Read the model definition and answer for the solid it produces. Units are mm, in the model's axes. Face numbers are marked on the shaded views. A direction names the side the tool comes from. Give positions to 0.01 mm unless a question says otherwise; leave off trailing zeros. Write each loop counter-clockwise with the first axis right and the second up, starting at its lowest first coordinate (ties: lowest second). Pieces come first, ordered by that corner, then holes. Notation, with made-up numbers: M 73.25,-14.75 L 108.25,-14.75 A23 ccw 108.25,20.25 Z; hole C -2.5,33 d1. An arc over 180 degrees is marked long. Use a Markdown table: item, result. Add a question column.
Item 1: A cutting plane is placed at C-C on x = 0. Count the separate pieces of the cut face and the enclosed holes in it, then the cut area to 3 significant figures.
Item 2: A cutting plane is placed at A-A on z = 47. Determine the outline of the cut face in (x, y), then the cut area to 3 significant figures.
Item 3: A cutting plane is placed at B-B on y = 0. Determine the outline of the cut face in (x, z).
Item 4: Consider probe 1 along Y at (x, z) = (0, -12.5); probe 2 along Y at (x, z) = (10.5, 41.5); probe 3 along Z at (x, y) = (-7, 9). Determine where each line is inside the solid, lowest interval first. Write a range as [from, to].
Item 5: For the marked faces 1 and 2, determine the directions among +Z, -Z, +X, -X, +Y, -Y from which every point of the face is accessible in a straight line to the end or side of a thin tool.
Item 6: The mould has two halves that part along Y. Classify the marked faces 3, 4 and 5: pulls with the +Y half, pulls with the -Y half, needs draft (parallel to the pull), parting line crosses it, or undercut.
Item 7: Given P1, Ø8, axis at x = 0, z = 63, coming from the +Y side; P2, Ø11.5, axis at x = -7.5, z = 46, coming from the -Y side; P3, Ø0.9, axis at y = 17, z = 46, coming from the +X side; P4, Ø19.5, axis at x = 0, y = 0, coming from the +Z side, each flat-ended and moving along its own axis, determine where each tip first touches the part or whether it passes through.
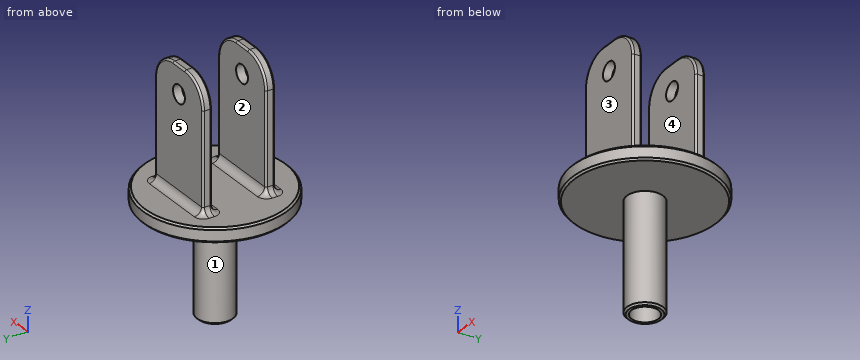
from build123d import *

# Parameters (mm, degrees)
SKETCH1_R            = 40
BOSS_EXTRUDE1_DEPTH  = 8
SKETCH2_W            = 40
SKETCH2_H            = 5
BOSS_EXTRUDE2_DEPTH  = 70
FILLET1_R            = 15
FILLET2_R            = 1
FILLET3_R            = 4
FILLET1_OF_MIRROR1_R = 15
FILLET2_OF_MIRROR1_R = 1
FILLET3_OF_MIRROR1_R = 4
SKETCH3_R            = 5
CUT_EXTRUDE1_DEPTH   = 107.226173873
SKETCH4_R            = 10
SKETCH4_R_2          = 7.5
BOSS_EXTRUDE3_DEPTH  = 60
CHAMFER1_SIZE        = 1
CHAMFER2_SIZE        = 1


with BuildPart() as part:
    # Sketch1 → Boss-Extrude1 (new body)
    with BuildSketch(Plane.XY):
        Circle(SKETCH1_R)
    extrude(amount=BOSS_EXTRUDE1_DEPTH)

    # Sketch2 → Boss-Extrude2 (add)
    with BuildSketch(Plane.XY.offset(8)):
        with Locations((0, 17.5)):
            Rectangle(SKETCH2_W, SKETCH2_H)
    boss_extrude2 = extrude(amount=BOSS_EXTRUDE2_DEPTH)

    # Fillet1
    fillet1_edges = [part.edges().sort_by_distance(p)[0] for p in [
        (-20, 17.5, 78),
        (20, 17.5, 78),
    ]]
    fillet(fillet1_edges, radius=FILLET1_R)

    # Fillet2
    fillet2_edges = [part.edges().sort_by_distance(p)[0] for p in [
        (0, 15, 78),
        (0, 20, 78),
        (-20, 20, 35.5),
        (20, 20, 35.5),
        (-15.606601718, 20, 73.606601718),
        (15.606601718, 20, 73.606601718),
        (20, 15, 35.5),
        (-20, 15, 35.5),
        (-15.606601718, 15, 73.606601718),
        (15.606601718, 15, 73.606601718),
    ]]
    fillet(fillet2_edges, radius=FILLET2_R)

    # Fillet3
    fillet3_edges = [part.edges().sort_by_distance(p)[0] for p in [
        (0, 20, 8),
        (20, 17.5, 8),
        (0, 15, 8),
        (-20, 17.5, 8),
        (19.707106781, 19.707106781, 8),
        (19.707106781, 15.292893219, 8),
        (-19.707106781, 19.707106781, 8),
        (-19.707106781, 15.292893219, 8),
    ]]
    fillet(fillet3_edges, radius=FILLET3_R)

    # Mirror1: Boss-Extrude2 across plane
    add(boss_extrude2.mirror(Plane.ZX))

    # Fillet1 of Mirror1
    fillet1_of_mirror1_edges = [part.edges().sort_by_distance(p)[0] for p in [
        (-20, -17.5, 78),
        (20, -17.5, 78),
    ]]
    fillet(fillet1_of_mirror1_edges, radius=FILLET1_OF_MIRROR1_R)

    # Fillet2 of Mirror1
    fillet2_of_mirror1_edges = [part.edges().sort_by_distance(p)[0] for p in [
        (0, -15, 78),
        (0, -20, 78),
        (-20, -20, 35.5),
        (20, -20, 35.5),
        (-15.606601718, -20, 73.606601718),
        (15.606601718, -20, 73.606601718),
        (20, -15, 35.5),
        (-20, -15, 35.5),
        (-15.606601718, -15, 73.606601718),
        (15.606601718, -15, 73.606601718),
    ]]
    fillet(fillet2_of_mirror1_edges, radius=FILLET2_OF_MIRROR1_R)

    # Fillet3 of Mirror1
    fillet3_of_mirror1_edges = [part.edges().sort_by_distance(p)[0] for p in [
        (0, -20, 8),
        (20, -17.5, 8),
        (0, -15, 8),
        (-20, -17.5, 8),
        (19.707106781, -19.707106781, 8),
        (19.707106781, -15.292893219, 8),
        (-19.707106781, -19.707106781, 8),
        (-19.707106781, -15.292893219, 8),
    ]]
    fillet(fillet3_of_mirror1_edges, radius=FILLET3_OF_MIRROR1_R)

    # Sketch3 → Cut-Extrude1 (cut, through all)
    with BuildSketch(Plane(origin=(0, 20, 0), x_dir=(1, 0, 0), z_dir=(0, 1, 0))):
        with Locations(Location((0, -63, 0), (0, 0, 180))):
            Circle(SKETCH3_R)
    extrude(amount=-CUT_EXTRUDE1_DEPTH, mode=Mode.SUBTRACT)

    # Sketch4 → Boss-Extrude3 (add)
    with BuildSketch(Plane(origin=(0, 0, 0), x_dir=(-1, 0, 0), z_dir=(0, 0, -1))):
        with Locations(Location((0, 0, 0), (0, 0, 180))):
            Circle(SKETCH4_R)
        with Locations(Location((0, 0, 0), (0, 0, 180))):
            Circle(SKETCH4_R_2, mode=Mode.SUBTRACT)
    extrude(amount=BOSS_EXTRUDE3_DEPTH)

    # Chamfer1
    chamfer1_edges = [part.edges().sort_by_distance(p)[0] for p in [
        (-10, 0, -60),
    ]]
    chamfer(chamfer1_edges, length=CHAMFER1_SIZE)

    # Chamfer2
    chamfer2_edges = [part.edges().sort_by_distance(p)[0] for p in [
        (-40, 0, 0),
        (-40, 0, 8),
    ]]
    chamfer(chamfer2_edges, length=CHAMFER2_SIZE)


solid = part.part
Filled in:
| question | item | result |
|---|---|---|
| 1 | separate pieces | 3 |
| 1 | enclosed holes | 0 |
| 1 | area | 1,550 mm² |
| 2 | outline | M -20,-19 A1 ccw -19,-20 L 19,-20 A1 ccw 20,-19 L 20,-16 A1 ccw 19,-15 L -19,-15 A1 ccw -20,-16 Z; M -20,16 A1 ccw -19,15 L 19,15 A1 ccw 20,16 L 20,19 A1 ccw 19,20 L -19,20 A1 ccw -20,19 Z |
| 2 | area | 398 mm² |
| 3 | outline | M -40,1 L -39,0 L -10,0 L -10,-59 L -9,-60 L -7.5,-60 L -7.5,0 L 7.5,0 L 7.5,-60 L 9,-60 L 10,-59 L 10,0 L 39,0 L 40,1 L 40,7 L 39,8 L -39,8 L -40,7 Z |
| 4 | probe 1 | [-10, -7.5], [7.5, 10] |
| 4 | probe 2 | [-20, -15], [15, 20] |
| 4 | probe 3 | [0, 8] |
| 5 | face 1 | -Z |
| 5 | face 2 | +Z, +X, -X |
| 6 | face 3 | pulls with the -Y half |
| 6 | face 4 | undercut |
| 6 | face 5 | pulls with the +Y half |
| 7 | P1 | through |
| 7 | P2 | y = -20 |
| 7 | P3 | x = 20 |
| 7 | P4 | z = 8 |
